For this review, take the finished solid that the model builds, in its own axes (mm). Face numbers are marked on the shaded views. A direction names the side the tool comes from. Round coordinates to 2 decimals unless told otherwise and drop trailing zeros. Write each loop counter-clockwise with the first axis right and the second up, starting at its lowest first coordinate (ties: lowest second). Pieces come first, ordered by that corner, then holes. Notation, with made-up numbers: M -21.5,43 L 3.5,43 A30 cw 3.5,74 Z; hole C -31,-5 d6. An arc over 180 degrees is marked long. Answer in a Markdown table with one row per item.
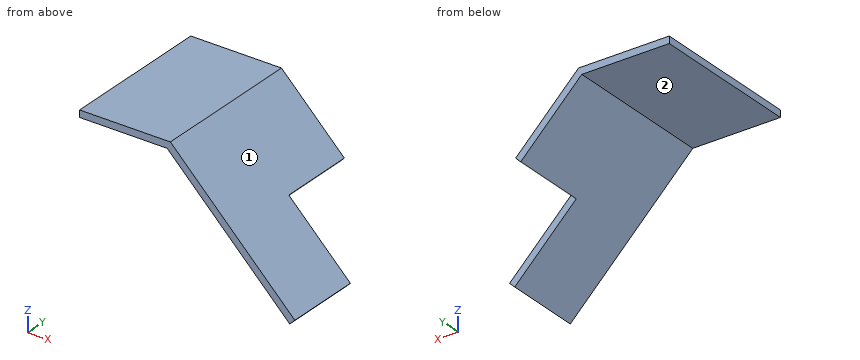
```python
from build123d import *

# Parameters (mm, degrees)
BOSS_EXTRUDE1_DEPTH = 7.62
CUT_EXTRUDE2_DEPTH  = 3.81


with BuildPart() as part:
    # Sketch1 → Boss-Extrude1 (new body)
    with BuildSketch(Plane(origin=(0, 0, 0), x_dir=(1, 0, 0), z_dir=(0, 1, 0))):
        Polygon((-0.253590848, 0), (-4.623419976, 0), (-4.623419976, -0.346366729), (-0.092515757, -0.346366729), (6.119785938, 5.855927972), (5.86619509, 6.109927972), align=None)
    extrude(amount=BOSS_EXTRUDE1_DEPTH)

    # Sketch3 → Cut-Extrude2 (cut)
    with BuildSketch(Plane(origin=(0, 7.62, 0), x_dir=(1, 0, 0), z_dir=(0, 1, 0))):
        Polygon((6.119785938, 5.855927972), (5.86619509, 6.109927972), (2.793767925, 3.042449981), (3.047358773, 2.788449981), align=None)
    extrude(amount=-CUT_EXTRUDE2_DEPTH, mode=Mode.SUBTRACT)


solid = part.part
```
Q1. Take a section at B-B (x = -2). State the section outline as (y, z) points.
Found:
| item | result |
|---|---|
| outline | M 0,0 L 7.62,0 L 7.62,0.35 L 0,0.35 Z |
Q2. Take a section at D-D (y = 1). State the section outline as (x, z) points.
Found:
| item | result |
|---|---|
| outline | M -4.62,0 L -0.25,0 L 5.87,-6.11 L 6.12,-5.86 L -0.09,0.35 L -4.62,0.35 Z |
Q3. Take a section at C-C (z = -0.5). State the section outline as (x, y) points, then the cut area to 3 significant figures.
Found:
| item | result |
|---|---|
| outline | M 0.25,0 L 0.76,0 L 0.76,7.62 L 0.25,7.62 Z |
| area | 3.87 mm² |
Q4. Take a section at A-A (y = 7). State the section outline as (x, z) points.
Found:
| item | result |
|---|---|
| outline | M -4.62,0 L -0.25,0 L 2.79,-3.04 L 3.05,-2.79 L -0.09,0.35 L -4.62,0.35 Z |
Q5. Insertion check: P1, Ø1.5, axis at x = -3, y = 2.5, coming from the -Z side; P2, Ø2, axis at x = 2.5, y = 5, coming from the -Z side; P3, Ø2.5, axis at x = 5, z = -4.5, coming from the +Y side. Each pin has a flat end and moves straight along its axis. Give the tip position at first contact, or say it passes through.
Found:
| item | result |
|---|---|
| P1 | z = 0 |
| P2 | z = -3.04 |
| P3 | y = 3.81 |
Q6. Machinability: for the marked faces 1 and 2, which of the approach directions +Z, -Z, +X, -X, +Y, -Y give a long, thin tool a straight path to every point of the face, cutting with its end or side? Answer none if there is none.
Found:
| item | result |
|---|---|
| face 1 | +Z, +X, +Y, -Y |
| face 2 | -Z, -X, +Y, -Y |
Q7. For probe 1 along Z at (x, y) = (-3.25, 1.75); probe 2 along X at (y, z) = (6.75, -1.25); probe 3 along X at (y, z) = (2.5, -3.5), list the stretches that pass through material, from the lowest coordinate up.
Found:
| item | result |
|---|---|
| probe 1 | 0 to 0.35 |
| probe 2 | 1 to 1.51 |
| probe 3 | 3.25 to 3.76 |
